Source: three-view drawing plus pictorial views. Frame: mm from the lowest corner of the part. A direction names the side the tool comes from. Give positions to 0.01 mm unless a question says otherwise; leave off trailing zeros. Order: outer loops, then holes, each group sorted by start corner. A loop starts at its lowest first (then second) coordinate and runs counter-clockwise, first axis right, second up. Notation, with made-up numbers: (57, 84.5) -> (68, 84.5) arc R15 cw to (68, 108.5) -> close; hole circle Ø3 at (51, 34). An arc over 180 degrees is marked (long way). Answer in a Markdown table with one row per item. Add a question column.
Q1. Cut plane C-C on x = 9. Return the cut outline in (y, z), and give its area (3 significant figures).
Q2. Cut plane B-B on y = 3.75. Return the cut outline in (x, z).
Q3. Cut plane A-A on z = 7.5. Return the cut outline in (x, y), and give its area (3 significant figures).
Q4. Line query: line 1 along X through (y, z) = (20.5, 7.5); line 2 along Y through (x, z) = (8.25, 4); line 3 along Y through (x, z) = (2.25, 4.75). Output: solid intervals per line, ascending. Write a range as from..to.
Q5. Cut plane D-D on x = 3. Return the cut outline in (y, z), and give its area (3 significant figures).
Q6. Pull-direction query (Z, two-part tool) for the marked faces 1, 2 and 3; classes: +Z half, -Z half, draft (parallel to the pull), parting line (faces both ways), or undercut.
Q7. Set-up query: the marked faces 4 and 5. Return all of +Z, -Z, +X, -X, +Y, -Y with unobstructed straight access to the full face (end or side cutting, diameter ignored); none if empty.
Q8. Contact query for flat-ended pins moving along their axis: P1, Ø2, axis at y = 3.5, z = 4.5, coming from the +X side; P2, Ø6, axis at y = 12.5, z = 12, coming from the -X side; P3, Ø3, axis at y = 26.5, z = 12, coming from the +X side. Output: stop coordinate, or through.
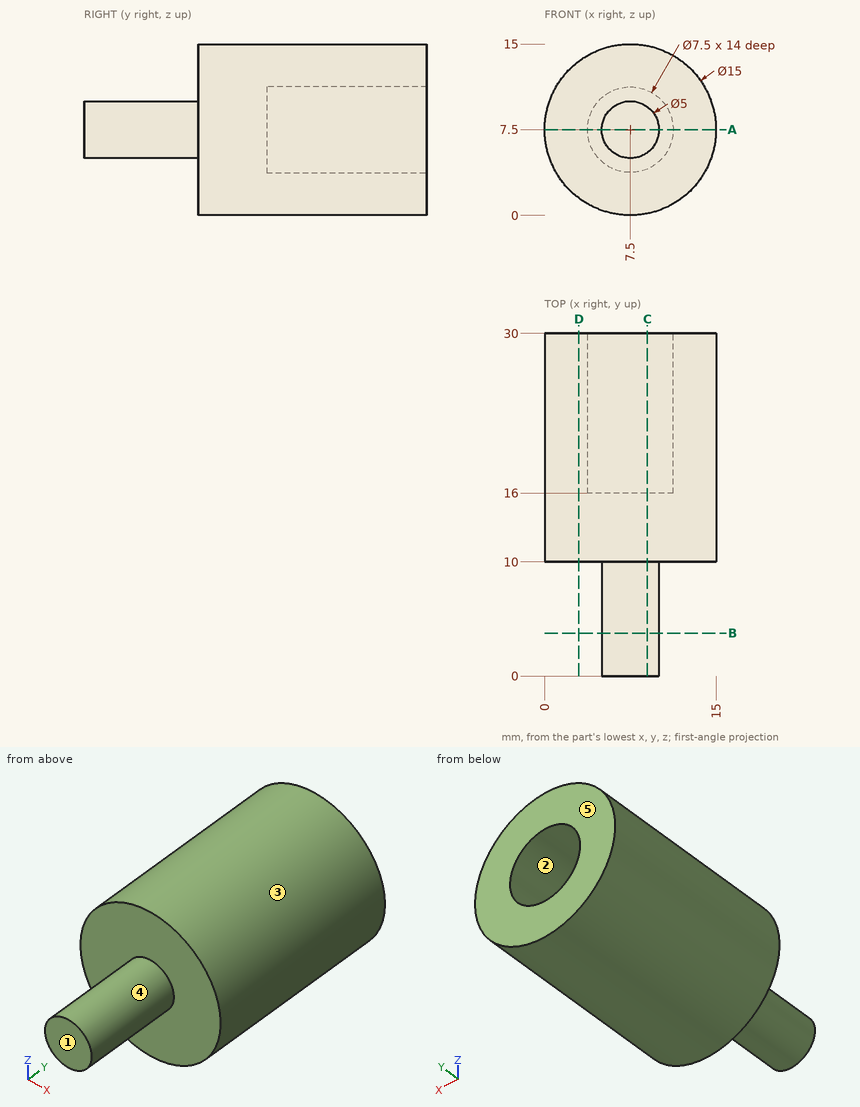
Completed:
| question | item | result |
|---|---|---|
| 1 | outline | (0, 5.5) -> (10, 5.5) -> (10, 0.15) -> (30, 0.15) -> (30, 4.06) -> (16, 4.06) -> (16, 10.94) -> (30, 10.94) -> (30, 14.85) -> (10, 14.85) -> (10, 9.5) -> (0, 9.5) -> close |
| 1 | area | 238 mm² |
| 2 | outline | circle Ø5 at (7.5, 7.5) |
| 3 | outline | (0, 10) -> (5, 10) -> (5, 0) -> (10, 0) -> (10, 10) -> (15, 10) -> (15, 30) -> (11.25, 30) -> (11.25, 16) -> (3.75, 16) -> (3.75, 30) -> (0, 30) -> close |
| 3 | area | 245 mm² |
| 4 | line 1 | x = 0..3.75, 11.25..15 |
| 4 | line 2 | y = 10..16 |
| 4 | line 3 | y = 10..30 |
| 5 | outline | (10, 1.5) -> (30, 1.5) -> (30, 13.5) -> (10, 13.5) -> close |
| 5 | area | 240 mm² |
| 6 | face 1 | draft |
| 6 | face 2 | undercut |
| 6 | face 3 | parting line |
| 7 | face 4 | -Y |
| 7 | face 5 | +Z, -Z, +X, -X, +Y |
| 8 | P1 | stops at x = 9 |
| 8 | P2 | stops at x = 0.15 |
| 8 | P3 | stops at x = 14.37 |
